For this review, use the dimensioned drawing (mm, ordinates from the lowest corner) and the shaded views. Give positions to 0.01 mm unless a question says otherwise; leave off trailing zeros. Order: outer loops, then holes, each group sorted by start corner. A loop starts at its lowest first (then second) coordinate and runs counter-clockwise, first axis right, second up. Notation, with made-up numbers: (-9, 34) - (35, 34) arc R26 cw to (35, 71) - close; hole circle Ø10 at (68.25, 6). An arc over 180 degrees is marked (long way). Use a Markdown table: item, result. Add a question column.
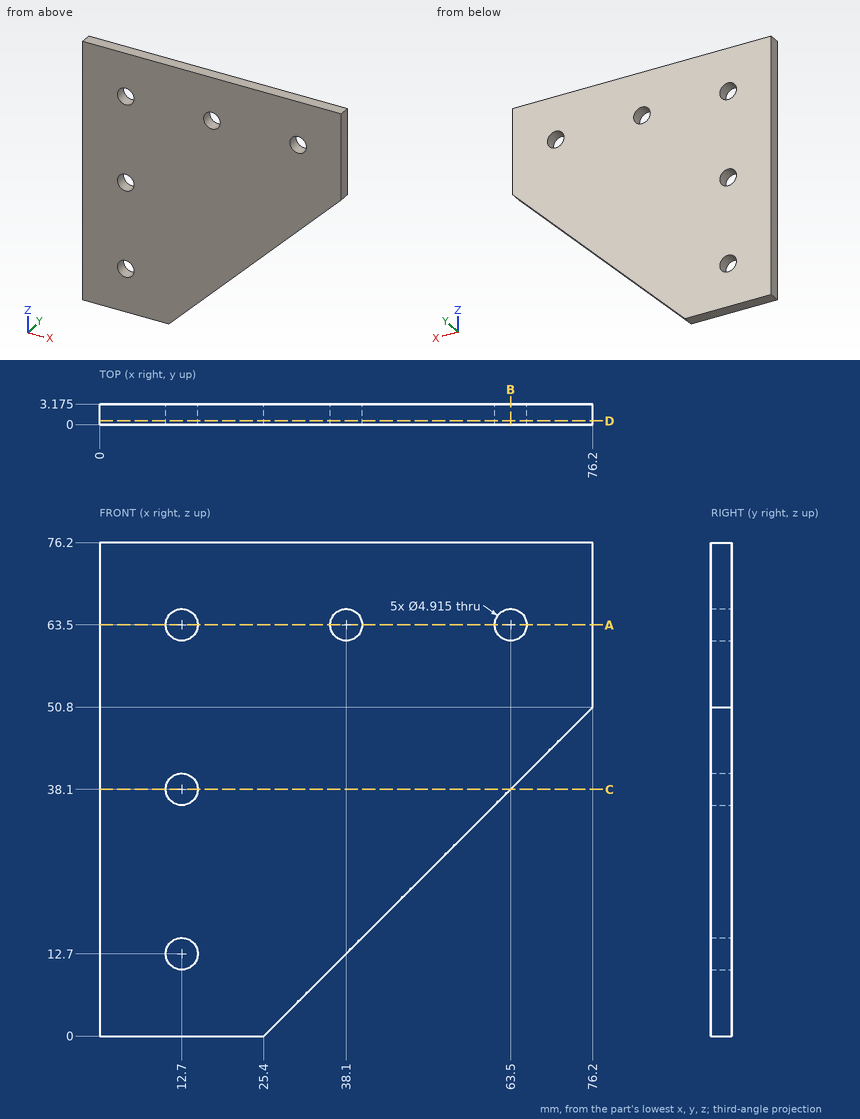
Q1. Clearance check with a flat-ended pin moving along its axis: P1, Ø1.5, axis at y = 1.5, z = 24.5, coming from the +X side. State where the tip first meets the part, or that it passes through.
Q2. We need section D-D (y = 0.55). Write out the cut boundary in (x, z) (1 decimal), plus the area to 3 significant figures.
Q3. We need section B-B (x = 63.5). Write out the cut boundary in (y, z) (1 decimal).
Q4. We need section C-C (z = 38.1). Write out the cut boundary in (x, y) (1 decimal).
Q5. Wall thickness on probe 1 along Z at (x, y) = (12.7, 2.1); probe 2 along X at (y, z) = (0.35, 63): over which ranges is each line inside the solid? List them lowest first.
Q6. We need section A-A (z = 63.5). Write out the cut boundary in (x, y) (1 decimal), plus the area to 3 significant figures.
Here are the results:
| question | item | result |
|---|---|---|
| 1 | P1 | x = 50.65 |
| 2 | outline | (0, 0) - (25.4, 0) - (76.2, 50.8) - (76.2, 76.2) - (0, 76.2) - close; hole circle Ø4.9 at (12.7, 12.7); hole circle Ø4.9 at (12.7, 38.1); hole circle Ø4.9 at (12.7, 63.5); hole circle Ø4.9 at (38.1, 63.5); hole circle Ø4.9 at (63.5, 63.5) |
| 2 | area | 4,420 mm2 |
| 3 | outline | (0, 38.1) - (3.2, 38.1) - (3.2, 61) - (0, 61) - close; (0, 66) - (3.2, 66) - (3.2, 76.2) - (0, 76.2) - close |
| 4 | outline | (0, 0) - (10.2, 0) - (10.2, 3.2) - (0, 3.2) - close; (15.2, 0) - (63.5, 0) - (63.5, 3.2) - (15.2, 3.2) - close |
| 5 | probe 1 | 0 to 10.24, 15.16 to 35.64, 40.56 to 61.04, 65.96 to 76.2 |
| 5 | probe 2 | 0 to 10.29, 15.11 to 35.69, 40.51 to 61.09, 65.91 to 76.2 |
| 6 | outline | (0, 0) - (10.2, 0) - (10.2, 3.2) - (0, 3.2) - close; (15.2, 0) - (35.6, 0) - (35.6, 3.2) - (15.2, 3.2) - close; (40.6, 0) - (61, 0) - (61, 3.2) - (40.6, 3.2) - close; (66, 0) - (76.2, 0) - (76.2, 3.2) - (66, 3.2) - close |
| 6 | area | 195 mm2 |
